Here's how the part is built. I have some questions about the finished solid (model axes, mm). Face numbers are marked on the shaded views. Round coordinates to 2 decimals unless told otherwise and drop trailing zeros. Write each loop counter-clockwise with the first axis right and the second up, starting at its lowest first coordinate (ties: lowest second). Pieces come first, ordered by that corner, then holes. Notation, with made-up numbers: (-2, 63) -> (38, 63) arc R30 ccw to (38, 99) -> close; hole circle Ø10 at (35, 78). An arc over 180 degrees is marked (long way). Put each result on its own line as item: value. Start each with the question number.
1) We'd pull the mould along X, two halves only. Please class the marked faces 1, 2 and 3: released by +X, released by -X, zero draft, split by the parting line, or undercut.
2) I want a section at B-B, the plane z = 1.3. Give the number of separate pieces and of enclosed holes in the cut face, then the cut area to 3 significant figures.
3) If I drill on line 1 along X through (y, z) = (0.1, 1.25); line 2 along X through (y, z) = (-0.85, 0.75); line 3 along Y through (x, z) = (-10.5, 0.65), over which ranges is the centre line in solid material (lowest first)? Write a range as [from, to].
4) I want a section at D-D, the plane y = -0.5. List the corners of the cut face in (x, z) for me, then the cut area to 4 significant figures.
5) I want a section at A-A, the plane x = 9.25. List the corners of the cut face in (y, z) for me, then the cut area to 3 significant figures.
6) I want a section at C-C, the plane y = 0.65. List the corners of the cut face in (x, z) for me.
from build123d import *

# Parameters (mm, degrees)
SKETCH1_W           = 25
SKETCH1_H           = 5
SKETCH1_R           = 1
BOSS_EXTRUDE1_DEPTH = 2
FILLET1_R           = 2.5


with BuildPart() as part:
    # Sketch1 → Boss-Extrude1 (new body)
    with BuildSketch(Plane.XY):
        Rectangle(SKETCH1_W, SKETCH1_H)
        with Locations((9.931042695, -0.076752974)):
            Circle(SKETCH1_R, mode=Mode.SUBTRACT)
        with Locations(Location((-9.931042695, -0.076752974, 0), (0, 0, 180))):
            Circle(SKETCH1_R, mode=Mode.SUBTRACT)
    extrude(amount=BOSS_EXTRUDE1_DEPTH)

    # Fillet1
    fillet1_edges = [part.edges().sort_by_distance(p)[0] for p in [
        (-12.5, -2.5, 1),
        (-12.5, 2.5, 1),
        (12.5, -2.5, 1),
        (12.5, 2.5, 1),
    ]]
    fillet(fillet1_edges, radius=FILLET1_R - 0.0001)  # a hair under: the kernel refuses the full size


solid = part.part
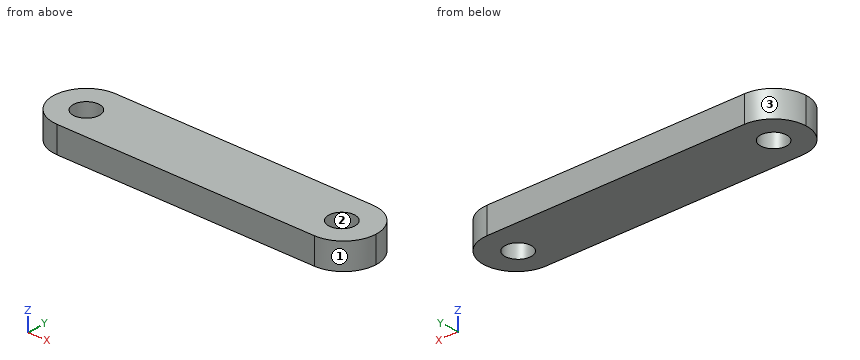
Findings:
1. face 1: released by +X
1. face 2: undercut
1. face 3: released by -X
2. separate pieces: 1
2. enclosed holes: 2
2. area: 113 mm2
3. line 1: x = [-12.5, -10.92], [-8.95, 8.95], [10.92, 12.5]
3. line 2: x = [-12.35, -10.57], [-9.3, 9.3], [10.57, 12.35]
3. line 3: y = [-2.45, -0.9], [0.75, 2.45]
4. outline: (-12.45, 0) -> (-10.84, 0) -> (-10.84, 2) -> (-12.45, 2) -> close; (-9.03, 0) -> (9.03, 0) -> (9.03, 2) -> (-9.03, 2) -> close; (10.84, 0) -> (12.45, 0) -> (12.45, 2) -> (10.84, 2) -> close
4. area: 42.55 mm2
5. outline: (-2.5, 0) -> (-0.81, 0) -> (-0.81, 2) -> (-2.5, 2) -> close; (0.66, 0) -> (2.5, 0) -> (2.5, 2) -> (0.66, 2) -> close
5. area: 7.07 mm2
6. outline: (-12.41, 0) -> (-10.62, 0) -> (-10.62, 2) -> (-12.41, 2) -> close; (-9.24, 0) -> (9.24, 0) -> (9.24, 2) -> (-9.24, 2) -> close; (10.62, 0) -> (12.41, 0) -> (12.41, 2) -> (10.62, 2) -> close
